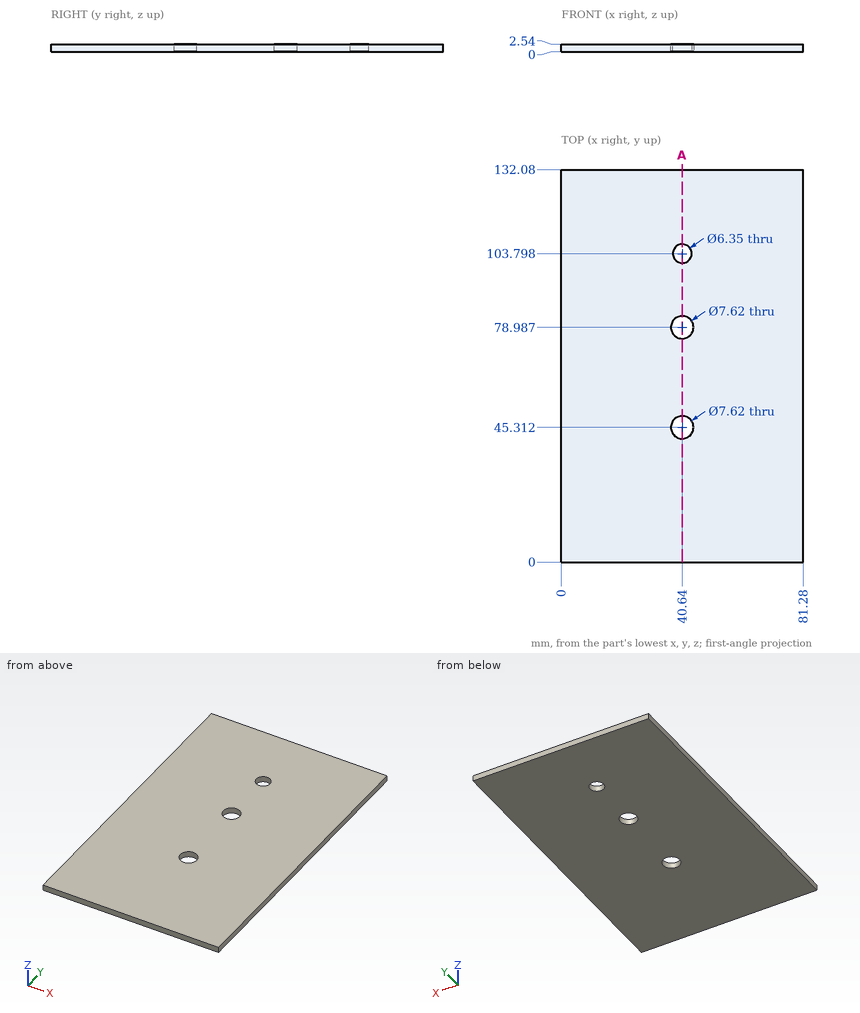
For this review, use the dimensioned drawing (mm, ordinates from the lowest corner) and the shaded views. Round coordinates to 2 decimals unless told otherwise and drop trailing zeros. Write each loop counter-clockwise with the first axis right and the second up, starting at its lowest first coordinate (ties: lowest second). Pieces come first, ordered by that corner, then holes. Notation, with made-up numbers: M 67,48 L 94,48 A25 ccw 94,75 Z; hole C -7,89.5 d4. An arc over 180 degrees is marked long. Answer as CSV lines item,"result". Start each with the question number.
Q1. Clearance check with flat-ended pins moving along their axes: P1, Ø8.5, axis at x = 40.64, y = 103.8, coming from the +Z side; P2, Ø4.5, axis at x = 40.64, y = 78.99, coming from the -Z side. State where each tip first meets the part, or that it passes through.
Q2. Consider section A-A, the plane x = 40.64. Give the boundary of the cut face in (y, z), then the cut area to 3 significant figures.
Q3. Wall thickness on line 1 along Y through (x, z) = (40.64, 1.7); line 2 along X through (y, z) = (45, 0.95); line 3 along Y through (x, z) = (41.5, 0.9) (1 decimal): over which ranges is each line inside the solid? List them lowest first.
Result set:
1,P1,"stops at z = 2.54"
1,P2,"passes through"
2,outline,"M 0,0 L 41.5,0 L 41.5,2.54 L 0,2.54 Z; M 49.12,0 L 75.18,0 L 75.18,2.54 L 49.12,2.54 Z; M 82.8,0 L 100.62,0 L 100.62,2.54 L 82.8,2.54 Z; M 106.97,0 L 132.08,0 L 132.08,2.54 L 106.97,2.54 Z"
2,area,"281 mm²"
3,line 1,"y = 0 to 41.5, 49.12 to 75.18, 82.8 to 100.62, 106.97 to 132.08"
3,line 2,"x = 0 to 36.84, 44.44 to 81.28"
3,line 3,"y = 0 to 41.6, 49 to 75.3, 82.7 to 100.7, 106.9 to 132.1"
